```python
from build123d import *

# Parameters (mm, degrees)
SKETCH_1_W               = 60
SKETCH_1_H               = 20
EXTRUDE_320_DEPTH        = 3
SKETCH_3_W               = 3
SKETCH_3_H               = 16
EXTRUDE_3_DEPTH          = 20
CUT_EXTRUDE_4_DEPTH      = 4
CUT_EXTRUDE_4_DEPTH_BACK = 58


with BuildPart() as part:
    # Эскиз1 → Extrude 320 (new body)
    with BuildSketch(Plane(origin=(0, 0, 0), x_dir=(1, 0, 0), z_dir=(0, 1, 0))):
        with Locations((30, 10)):
            Rectangle(SKETCH_1_W, SKETCH_1_H)
    extrude(amount=EXTRUDE_320_DEPTH)

    # Эскиз3 → Бобышка-Вытянуть3 (add)
    with BuildSketch(Plane(origin=(0, 3, 0), x_dir=(1, 0, 0), z_dir=(0, 1, 0))):
        with Locations((4.5, 10)):
            Rectangle(SKETCH_3_W, SKETCH_3_H)
        with Locations((55.5, 10)):
            Rectangle(SKETCH_3_W, SKETCH_3_H)
    extrude(amount=EXTRUDE_3_DEPTH)

    # Эскиз13 → Вырез-Вытянуть4 (cut, two sides)
    with BuildSketch(Plane(origin=(57, 0, 0), x_dir=(0, 0, -1), z_dir=(1, 0, 0))) as cut_extrude_4_sk:
        Polygon((7, 23), (10, 17.110151736), (13, 23), align=None)
    extrude(amount=CUT_EXTRUDE_4_DEPTH, mode=Mode.SUBTRACT)
    extrude(cut_extrude_4_sk.sketch, amount=-CUT_EXTRUDE_4_DEPTH_BACK, mode=Mode.SUBTRACT)


solid = part.part
```
Model file for the job. Use its own axes, mm. A direction names the side the tool comes from. Give positions to 0.01 mm unless a question says otherwise; leave off trailing zeros. Order: outer loops, then holes, each group sorted by start corner. A loop starts at its lowest first (then second) coordinate and runs counter-clockwise, first axis right, second up.
1) 3-axis set-ups, long thin cutter, end or side, ignore diameter. For faces 1 (the flat face through (55.521, 20.014, -11.479)), 2 (the flat face through (6, 13, -10)), 3 (the flat face through (4, 13, -18)), 4 (the flat face through (57, 13, -10)): which of +Z, -Z, +X, -X, +Y, -Y reach the whole face in a straight line?
2) Saw through at B-B, the plane y = 20. Write the cut outline in (x, z), then the cut area to 3 significant figures.
3) Saw through at D-D, the plane x = 32. Write the cut outline in (y, z).
4) Saw through at C-C, the plane z = -3.5. Write the cut outline in (x, y), then the cut area to 3 significant figures.
5) Wall check: probe 1 along X at (y, z) = (18, -8.5); probe 2 along Y at (x, z) = (21, -1.75); probe 3 along Z at (x, y) = (4, 18.25). Give the ranges that are in metal, low to high.
6) Mould opens along Z. For faces 5 (the flat face through (3, 13, -10)), 6 (the flat face through (55.521, 20.096, -8.479)), 7 (the flat face through (55, 13, -2)) say: +Z half, -Z half, draft (parallel to the pull), parting line (faces both ways), or undercut.
7) Saw through at A-A, the plane y = 9.75. Write the cut outline in (x, z), then the cut area to 3 significant figures.
8) Pin check, flat tips, straight feed: pin 1 (10 mm diameter, centred on x = 19.5, z = -6.5, fed in from +Y); pin 2 (10 mm diameter, centred on y = 5, z = -3.5, fed in from -X); pin 3 (1 mm diameter, centred on y = 15, z = -16, fed in from -X); pin 4 (0.9 mm diameter, centred on x = 55.5, y = 12.5, fed in from +Z). Stop position of each tip, or through.
Computed:
1. face 1: +X, -X, +Y
1. face 2: +Z, -Z, +Y
1. face 3: -Z, +X, -X, +Y
1. face 4: +Z, -Z, +X, +Y
2. outline: (3, -18) - (6, -18) - (6, -11.47) - (3, -11.47) - close; (3, -8.53) - (6, -8.53) - (6, -2) - (3, -2) - close; (54, -18) - (57, -18) - (57, -11.47) - (54, -11.47) - close; (54, -8.53) - (57, -8.53) - (57, -2) - (54, -2) - close
2. area: 78.3 mm2
3. outline: (0, -20) - (3, -20) - (3, 0) - (0, 0) - close
4. outline: (0, 0) - (60, 0) - (60, 3) - (57, 3) - (57, 23) - (54, 23) - (54, 3) - (6, 3) - (6, 23) - (3, 23) - (3, 3) - (0, 3) - close
4. area: 300 mm2
5. probe 1: x = 3 to 6, 54 to 57
5. probe 2: y = 0 to 3
5. probe 3: z = -18 to -10.58, -9.42 to -2
6. face 5: draft
6. face 6: undercut
6. face 7: +Z half
7. outline: (3, -18) - (6, -18) - (6, -2) - (3, -2) - close; (54, -18) - (57, -18) - (57, -2) - (54, -2) - close
7. area: 96.0 mm2
8. pin 1: stops at y = 3
8. pin 2: stops at x = 0
8. pin 3: stops at x = 3
8. pin 4: stops at z = -2
